Design review of the part built by this model. Coordinates are the model's own, in mm. Give positions to 0.01 mm unless a question says otherwise; leave off trailing zeros. Loops run counter-clockwise (first coordinate to the right, second up) from the corner with the lowest first, then second, coordinate; pieces in that order, holes last. Notation, with made-up numbers: (-19, 11.5) -> (21, 11.5) arc R28 ccw to (21, 36.5) -> close; hole circle Ø10 at (2.25, -15). An arc over 180 degrees is marked (long way). Answer as CSV lines item,"result".
Autodesk Inventor part; units mm, degrees
ref_plane "YZ Plane" through (0, 0, 0) normal (1, 0, 0) x (0, 1, 0)
ref_plane "XZ Plane" through (0, 0, 0) normal (0, 1, 0) x (-1, 0, 0)
ref_plane "XY Plane" through (0, 0, 0) normal (0, 0, 1) x (1, 0, 0)
sketch "Sketch1" plane through (0, 0, 0) normal (0, 1, 0) x (-1, 0, 0)
  line L0 (-12, -3) -> (12, -3)
  line L1 (12, -3) -> (12, 3)
  line L2 (12, 3) -> (-12, 3)
  line L3 (-12, 3) -> (-12, -3)
  line L4 (-12, -3) -> (12, 3) construction
  line L5 (12, -3) -> (-12, 3) construction
  circle A0 centre (12, 0) radius 3
  circle A1 centre (-12, 0) radius 3
  point P0 (0, 0)
  dimension "d0" = 24
  dimension "d1" = 6
  dimension "d2" = 6
  dimension "d3" = 6
extrude "Extrusion1" add sketch "Sketch1" along normal blind 2
sketch "Sketch2" plane through (0, 2, 0) normal (0, 1, 0) x (1, 0, 0)
  arc A0 (12, -3) -> (12, 3) centre (12, 0) ccw
  arc A1 (-12, 3) -> (-12, -3) centre (-12, 0) ccw
  circle A2 centre (-12, 0) radius 1
  circle A3 centre (12, 0) radius 1.5
  circle A4 centre (-12, 0) radius 1.5
  point P0 (0, 0)
  dimension "d6" = 2
  dimension "d7" = 3
  dimension "d8" = 3
extrude "Extrusion2" cut sketch "Sketch2" against normal blind 2 contours A2 | A3 | A4
sketch "Sketch3" plane through (0, 0, 0) normal (0, -1, 0) x (1, 0, 0)
  circle A0 centre (12, 0) radius 1.5
  circle A1 centre (-12, 0) radius 1.5
  arc A2 (12, -3) -> (12, 3) centre (12, 0) ccw
  arc A3 (-12, 3) -> (-12, -3) centre (-12, 0) ccw
  circle A4 centre (-12, 0) radius 0.005
  circle A5 centre (12, 0) radius 0.005
  point P0 (0, 0)
  dimension "d11" = 0.01
  dimension "d12" = 0.01
extrude "Extrusion3" add sketch "Sketch3" against normal blind 2
sketch "Sketch4" plane through (0, 0, 0) normal (0, -1, 0) x (1, 0, 0)
  arc A0 (12, -3) -> (12, 3) centre (12, 0) ccw
  arc A1 (-12, 3) -> (-12, -3) centre (-12, 0) ccw
  circle A2 centre (-12, 0) radius 0.05
  circle A3 centre (12, 0) radius 0.05
  point P0 (0, 0)
  dimension "d15" = 0.1
  dimension "d16" = 0.1
extrude "Extrusion4" cut sketch "Sketch4" against normal blind 2
properties part number "tahlo5_sablona"
Q1. To check wall thickness, follow probe 1 along X at (y, z) = (1.2, 0.1); probe 2 along Z at (x, y) = (13.25, 0.1); probe 3 along X at (y, z) = (1.35, 1.8). State the ranges of each line that lie inside material, in increasing order. Write a range as from..to.
Filled sheet:
probe 1,"x = -15..15"
probe 2,"z = -2.73..2.73"
probe 3,"x = -14.4..14.4"
Q2. We need section A-A, the plane y = 0.5. State the section outline as (x, z) points, and give its area (3 significant figures).
Filled sheet:
outline,"(-12, -3) -> (12, -3) arc R3 ccw to (12, 3) -> (-12, 3) arc R3 ccw to start; hole circle Ø0.1 at (-12, 0); hole circle Ø0.1 at (12, 0)"
area,"172 mm^2"
Q3. We need section B-B, the plane z = -2.6. State the section outline as (x, y) points, and give its area (3 significant figures).
Filled sheet:
outline,"(-13.5, 0) -> (13.5, 0) -> (13.5, 2) -> (-13.5, 2) -> close"
area,"54.0 mm^2"
Q4. We need section C-C, the plane z = 1.4. State the section outline as (x, y) points.
Filled sheet:
outline,"(-14.65, 0) -> (14.65, 0) -> (14.65, 2) -> (-14.65, 2) -> close"
